Build history of the part. All positions in model axes, mm. A direction names the side the tool comes from. Give positions to 0.01 mm unless a question says otherwise; leave off trailing zeros. Order: outer loops, then holes, each group sorted by start corner. A loop starts at its lowest first (then second) coordinate and runs counter-clockwise, first axis right, second up. Notation, with made-up numbers: M 52.5,-40 L 62.5,-40 A25 cw 62.5,-25 Z; hole C 88,9 d1. An arc over 180 degrees is marked long. Answer as CSV lines item,"result".
Autodesk Inventor part; units mm, degrees
ref_plane "YZ Plane" through (0, 0, 0) normal (1, 0, 0) x (0, 1, 0)
ref_plane "XZ Plane" through (0, 0, 0) normal (0, 1, 0) x (-1, 0, 0)
ref_plane "XY Plane" through (0, 0, 0) normal (0, 0, 1) x (1, 0, 0)
ref_plane "Work Plane2" through (0, 0, 0) normal (0, 0, 1) x (1, 0, 0)
sketch "Sketch1" plane through (0, 0, 0) normal (0, 0, 1) x (1, 0, 0)
  line L0 (22.4943, 24.3103) -> (33.4943, 24.3103)
  line L1 (33.4943, 24.3103) -> (33.4943, 9.3103)
  line L2 (33.4943, 9.3103) -> (22.4943, 9.3103)
  line L3 (22.4943, 9.3103) -> (22.4943, 24.3103)
  point P0 (0, 0)
  dimension "d0" = 11
  dimension "d2" = 15
extrude "Extrusion1" add sketch "Sketch1" along normal blind 5.6
chamfer "Chamfer1" distance 2 angle 45 2 edges at (27.9943, 9.3103, 0) (27.9943, 24.3103, 0)
shell "Shell1" thickness 0.3 removed faces 1 at (33.4943, 18.6436, 3.7333)
sketch "Sketch2" plane through (22.7943, 9.6103, 5.3) normal (1, 0, 0) x (0, 0, -1)
  line L0 (3.1757, 14.4) -> (0, 14.4)
  line L1 (0, 14.4) -> (0, 0)
  line L2 (3.1757, 0) -> (0, 0)
  line L3 (2.6, 12.4) -> (1.6, 12.4)
  line L4 (1.6, 12.4) -> (1.6, 2)
  line L5 (1.6, 2) -> (2.6, 2)
  line L6 (2.6, 2) -> (2.6, 12.4)
  point P0 (5.3, -9.6103)
  dimension "d9" = 1
  dimension "d12" = 2
  dimension "d13" = 2
  dimension "d14" = 1.6
extrude "Extrusion2" add sketch "Sketch2" along normal up to surface (10.7 mm away)
properties part number "nanopc_t4_hdmi"
Item 1: Pull direction Y, two halves, no side cores. Call faces 1 (the flat face through (28, 17, 3.7)), 2 (the flat face through (27.92, 10.32, 0.99)), 3 (the flat face through (28, 17, 0)): released by +Y, released by -Y, zero draft, split by the parting line, or undercut.
Geometry says:
face 1,"undercut"
face 2,"released by -Y"
face 3,"zero draft"
Item 2: 3-axis set-ups, long thin cutter, end or side, ignore diameter. For faces 4 (the flat face through (28, 9.31, 4)), 5 (the flat face through (28, 9.61, 4)): which of +Z, -Z, +X, -X, +Y, -Y reach the whole face in a straight line?
Geometry says:
face 4,"+Z, -Z, +X, -X, -Y"
face 5,"+X"
Item 3: Band-saw the part on A-A (x = 24.75). Give the cut face in (y, z).
Geometry says:
outline,"M 9.31,2 L 11.31,0 L 22.31,0 L 24.31,2 L 24.31,5.6 L 9.31,5.6 Z; M 11.61,2.7 L 22.01,2.7 L 22.01,3.7 L 11.61,3.7 Z; hole M 9.61,2.12 L 11.43,0.3 L 22.19,0.3 L 24.01,2.12 L 24.01,5.3 L 9.61,5.3 Z"
Item 4: Band-saw the part on B-B (z = 4.9). Give the cut face in (x, y).
Geometry says:
outline,"M 22.49,9.31 L 33.49,9.31 L 33.49,9.61 L 22.79,9.61 L 22.79,24.01 L 33.49,24.01 L 33.49,24.31 L 22.49,24.31 Z"
Item 5: Band-saw the part on C-C (y = 13). Give the cut face in (x, z), and give its area (3 significant figures).
Geometry says:
outline,"M 22.49,0 L 33.49,0 L 33.49,0.3 L 22.79,0.3 L 22.79,2.7 L 33.49,2.7 L 33.49,3.7 L 22.79,3.7 L 22.79,5.3 L 33.49,5.3 L 33.49,5.6 L 22.49,5.6 Z"
area,"18.8 mm2"
Item 6: Band-saw the part on D-D (z = 1.2). Give the cut face in (x, y), and give its area (3 significant figures).
Geometry says:
outline,"M 22.49,10.11 L 33.49,10.11 L 33.49,10.53 L 22.79,10.53 L 22.79,23.09 L 33.49,23.09 L 33.49,23.51 L 22.49,23.51 Z"
area,"13.1 mm2"
Item 7: Probe line 1 along Z through (x, y) = (28, 21.5); line 2 along Y through (x, z) = (29.5, 3.65); line 3 along Y through (x, z) = (27.5, 2.4). List the from-to ranges inside material, lowest first. Write a range as from..to.
Geometry says:
line 1,"z = 0..0.3, 2.7..3.7, 5.3..5.6"
line 2,"y = 9.31..9.61, 11.61..22.01, 24.01..24.31"
line 3,"y = 9.31..9.61, 24.01..24.31"
